Design review of the part built by this model. Coordinates are the model's own, in mm. Round coordinates to 2 decimals unless told otherwise and drop trailing zeros. Order: outer loops, then holes, each group sorted by start corner. A loop starts at its lowest first (then second) coordinate and runs counter-clockwise, first axis right, second up.
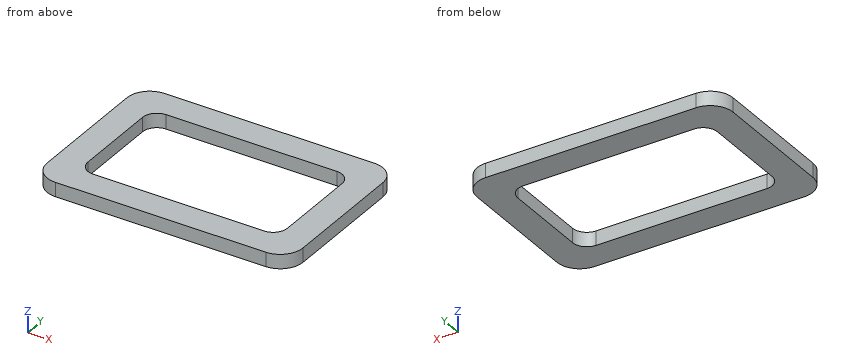
from build123d import *

# Parameters (mm, degrees)
BOSS_EXTRUDE1_DEPTH = 5
FILLET1_R           = 8
FILLET3_R           = 5


with BuildPart() as part:
    # Sketch1 → Boss-Extrude1 (new body)
    with BuildSketch(Plane.XY):
        Polygon((49.511947656, -13.648927203), (4.611947656, -13.648927203), (4.611947656, 46.251072797), (49.511947656, 46.251072797), (49.511947656, 36.351072797), (14.511947656, 36.351072797), (14.511947656, -3.748927203), (49.511947656, -3.748927203), align=None)
    boss_extrude1 = extrude(amount=BOSS_EXTRUDE1_DEPTH)

    # Mirror1: Boss-Extrude1 across plane
    add(boss_extrude1.mirror(Plane(origin=(49.511947656, 0, 0), x_dir=(0, 0, 1), z_dir=(1, 0, 0))))

    # Fillet1
    fillet1_edges = [part.edges().sort_by_distance(p)[0] for p in [
        (4.611947656, -13.648927203, 2.5),
        (4.611947656, 46.251072797, 2.5),
        (94.411947656, -13.648927203, 2.5),
        (94.411947656, 46.251072797, 2.5),
    ]]
    fillet(fillet1_edges, radius=FILLET1_R)

    # Fillet3
    fillet3_edges = [part.edges().sort_by_distance(p)[0] for p in [
        (14.511947656, 36.351072797, 2.5),
        (14.511947656, -3.748927203, 2.5),
        (84.511947656, 36.351072797, 2.5),
        (84.511947656, -3.748927203, 2.5),
    ]]
    fillet(fillet3_edges, radius=FILLET3_R)


solid = part.part
1) Take a section at A-A on x = 61. Give the boundary of the cut face in (y, z), plus the area to 3 significant figures.
Results:
outline: (-13.65, 0) - (-3.75, 0) - (-3.75, 5) - (-13.65, 5) - close; (36.35, 0) - (46.25, 0) - (46.25, 5) - (36.35, 5) - close
area: 99.0 mm2
2) Take a section at C-C on y = 24. Give the boundary of the cut face in (x, z), plus the area to 3 significant figures.
Results:
outline: (4.61, 0) - (14.51, 0) - (14.51, 5) - (4.61, 5) - close; (84.51, 0) - (94.41, 0) - (94.41, 5) - (84.51, 5) - close
area: 99.0 mm2
3) Take a section at B-B on z = 2.75. Give the boundary of the cut face in (x, y).
Results:
outline: (4.61, -5.65) arc R8 ccw to (12.61, -13.65) - (86.41, -13.65) arc R8 ccw to (94.41, -5.65) - (94.41, 38.25) arc R8 ccw to (86.41, 46.25) - (12.61, 46.25) arc R8 ccw to (4.61, 38.25) - close; hole (14.51, 1.25) arc R5 ccw to (19.51, -3.75) - (79.51, -3.75) arc R5 ccw to (84.51, 1.25) - (84.51, 31.35) arc R5 ccw to (79.51, 36.35) - (19.51, 36.35) arc R5 ccw to (14.51, 31.35) - close
4) To check wall thickness, follow line 1 along Y through (x, z) = (68, 0.7); line 2 along X through (y, z) = (3, 2.5); line 3 along Y through (x, z) = (16.5, 1.1). State the ranges of each line that lie inside material, in increasing order.
Results:
line 1: y = -13.65 to -3.75, 36.35 to 46.25
line 2: x = 4.61 to 14.51, 84.51 to 94.41
line 3: y = -13.65 to -2.74, 35.34 to 46.25
